Part model, mm, in its own coordinate system. Face numbers are marked on the shaded views. A direction names the side the tool comes from. Round coordinates to 2 decimals unless told otherwise and drop trailing zeros. Loops run counter-clockwise (first coordinate to the right, second up) from the corner with the lowest first, then second, coordinate; pieces in that order, holes last. Notation, with made-up numbers: (68, -35.75) - (125, -35.75) arc R16 cw to (125, -17.75) - close; hole circle Ø11 at (6.5, -25.5). An arc over 180 degrees is marked (long way). Put each result on its own line as item: value.
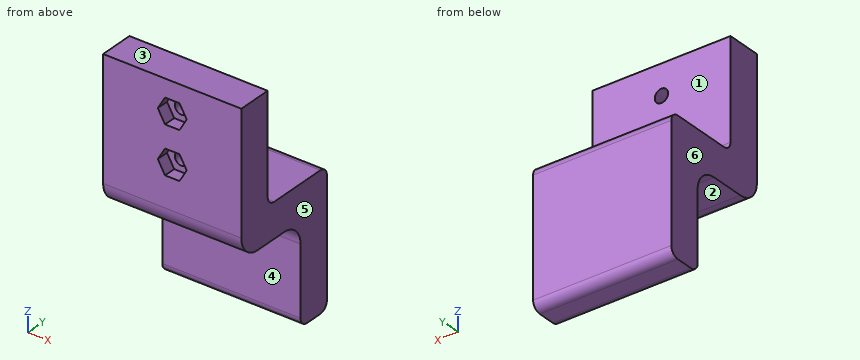
from build123d import *

# Parameters (mm, degrees)
SKETCH_1_W              = 32
SKETCH_1_H              = 32.917571433
EXTRUDE_1_DEPTH         = 8
CUT_EXTRUDE_1_DEPTH     = 2.8
CUT_EXTRUDE_2_DEPTH     = 2.8
HOLE_WIZARD_3_1_3_1_1_D = 3.1
SKETCH_9_W              = 8
SKETCH_9_H              = 18
EXTRUDE_3_DEPTH         = 32
SKETCH_10_W             = 23
SKETCH_10_H             = 8
EXTRUDE_4_DEPTH         = 32
FILLET_1_R              = 2
FILLET_2_R              = 2
FILLET_3_R              = 5


with BuildPart() as part:
    # 草图1 → 凸台-拉伸1 (new body)
    with BuildSketch(Plane.XZ):
        with Locations((0, 6.041214283)):
            Rectangle(SKETCH_1_W, SKETCH_1_H)
    extrude(amount=-EXTRUDE_1_DEPTH)

    # 草图2 → 切除-拉伸1 (cut)
    with BuildSketch(Plane.XZ):
        Polygon((-1.674315781, 18.4), (-3.348631561, 15.5), (-1.674315781, 12.6), (1.674315781, 12.6), (3.348631561, 15.5), (1.674315781, 18.4), align=None)
    extrude(amount=-CUT_EXTRUDE_1_DEPTH, mode=Mode.SUBTRACT)

    # 草图3 → 切除-拉伸2 (cut)
    with BuildSketch(Plane.XZ):
        Polygon((1.674315781, 7.4), (-1.674315781, 7.4), (-3.348631561, 4.5), (-1.674315781, 1.6), (1.674315781, 1.6), (3.348631561, 4.5), align=None)
    extrude(amount=-CUT_EXTRUDE_2_DEPTH, mode=Mode.SUBTRACT)

    # Ø3.1 (3.1) 直径孔1 (through all)
    with Locations(Plane(origin=(0, 2.8, 0), x_dir=(-1, 0, 0), z_dir=(0, -1, 0))):
        with Locations((0, -4.5), (0, -15.5)):
            Hole(HOLE_WIZARD_3_1_3_1_1_D / 2)

    # 草图9 → 凸台-拉伸3 (add)
    with BuildSketch(Plane(origin=(16, 0, 0), x_dir=(0, 0, -1), z_dir=(1, 0, 0))):
        with Locations((6.417571433, 17)):
            Rectangle(SKETCH_9_W, SKETCH_9_H)
    extrude(amount=-EXTRUDE_3_DEPTH)

    # 草图10 → 凸台-拉伸4 (add)
    with BuildSketch(Plane(origin=(16, 0, 0), x_dir=(0, 0, -1), z_dir=(1, 0, 0))):
        with Locations((21.917571433, 22)):
            Rectangle(SKETCH_10_W, SKETCH_10_H)
    extrude(amount=-EXTRUDE_4_DEPTH)

    # 圆角1
    fillet_1_edges = [part.edges().sort_by_distance(p)[0] for p in [
        (0, 8, -2.417571433),
        (0, 26, -2.417571433),
    ]]
    fillet(fillet_1_edges, radius=FILLET_1_R)

    # 圆角2
    fillet_2_edges = [part.edges().sort_by_distance(p)[0] for p in [
        (0, 26, -33.417571433),
        (0, 18, -33.417571433),
    ]]
    fillet(fillet_2_edges, radius=FILLET_2_R)

    # 圆角3
    fillet_3_edges = [part.edges().sort_by_distance(p)[0] for p in [
        (0, 0, -10.417571433),
        (0, 18, -10.417571433),
    ]]
    fillet(fillet_3_edges, radius=FILLET_3_R)


solid = part.part
1. Band-saw the part on C-C (x = 9). List the corners of the cut face in (y, z), plus the area to 3 significant figures.
A:
outline: (0, -5.42) arc R5 ccw to (5, -10.42) - (13, -10.42) arc R5 cw to (18, -15.42) - (18, -31.42) arc R2 ccw to (20, -33.42) - (24, -33.42) arc R2 ccw to (26, -31.42) - (26, -4.42) arc R2 ccw to (24, -2.42) - (10, -2.42) arc R2 cw to (8, -0.42) - (8, 22.5) - (0, 22.5) - close
area: 590 mm²
2. Tool access for the marked faces 1, 2 and 3: list every direction of +Z, -Z, +X, -X, +Y, -Y with a clear straight run to the whole face (end or side of a thin tool).
A:
face 1: +Z, +X, -X, +Y
face 2: -Z, +X, -X, -Y
face 3: +Z, +X, -X, +Y, -Y
3. Two-plate mould, pull along X, no slides. Class the marked faces 4, 5 and 6: pulls with the +X half, pulls with the -X half, needs draft (parallel to the pull), parting line crosses it, or undercut.
A:
face 4: needs draft
face 5: pulls with the +X half
face 6: pulls with the -X half
4. Band-saw the part on B-B (y = 6.25). List the corners of the cut face in (x, z).
A:
outline: (-16, -10.42) - (16, -10.42) - (16, 22.5) - (-16, 22.5) - close; hole circle Ø3.1 at (0, 4.5); hole circle Ø3.1 at (0, 15.5)
5. Band-saw the part on D-D (z = 19.5). List the corners of the cut face in (x, y), plus the area to 3 significant figures.
A:
outline: (-16, 0) - (16, 0) - (16, 8) - (-16, 8) - close
area: 256 mm²
6. Pin check, flat tips, straight feed: P1, Ø4.5, axis at x = 0, z = 15, coming from the -Y side; P2, Ø9, axis at x = 7, y = 8, coming from the -Z side; P3, Ø1, axis at x = -9.5, y = 10.5, coming from the +Z side. Stop position of each tip, or through.
A:
P1: stops at y = 2.8
P2: stops at z = -10.42
P3: stops at z = -2.42
7. Band-saw the part on A-A (x = 0). Give the number of separate pieces and of enclosed holes in the cut face, plus the area to 3 significant figures.
A:
separate pieces: 3
enclosed holes: 0
area: 525 mm²
8. Probe line 1 along Z through (x, y) = (0, 6.05); line 2 along X through (y, z) = (4.7, 4.5); line 3 along Z through (x, y) = (0, 4). List the from-to ranges inside material, lowest first. Write a range as [from, to].
A:
line 1: z = [-10.42, 2.95], [6.05, 13.95], [17.05, 22.5]
line 2: x = [-16, -1.55], [1.55, 16]
line 3: z = [-10.32, 2.95], [6.05, 13.95], [17.05, 22.5]
